Geometry check sheet. Reference: the model listing, model coordinates, mm. A direction names the side the tool comes from. Round coordinates to 2 decimals unless told otherwise and drop trailing zeros. Loops run counter-clockwise (first coordinate to the right, second up) from the corner with the lowest first, then second, coordinate; pieces in that order, holes last. Notation, with made-up numbers: M 78,35.5 L 132,35.5 A17 cw 132,66.5 Z; hole C 82.25,17.5 d1. An arc over 180 degrees is marked long. Use one line per item in the form item = value. Start each with the question number.
1. Material ranges on line 1 (Z direction, x = 10.75, y = -33); line 2 (X direction, y = 35.5, z = 5.75); line 3 (Z direction, x = -11.9, y = 31.75), recorded low to high.
2. Go/stop test with flat-tipped pins: pin 1 (1.5 mm diameter, centred on x = -6, y = -5.5, fed in from -Z); pin 2 (4 mm diameter, centred on y = 24, z = 4.5, fed in from +X). Record where each tip stops, or that it passes through.
3. Cross-section at D-D (z = -9.5). Record the boundary of the cut face in (x, y), then the cut area to 3 significant figures.
4. Cross-section at C-C (y = -19.5). Record the boundary of the cut face in (x, z) (1 decimal).
5. Cross-section at A-A (y = 31.75). Record the boundary of the cut face in (x, z) (1 decimal), then the cut area to 3 significant figures.
6. Draft check along Y on faces 3 (the flat face through (-12, 38.1, 4)), 4 (the cylindrical face through (-2.65, 1.43, 10.5)), 5 (the flat face through (-12, 1, -13.288)). Enter one of: pulls with the +Y half, pulls with the -Y half, needs draft (parallel to the pull), parting line crosses it, or undercut.
7. Cross-section at B-B (z = -4.25). Record the boundary of the cut face in (x, y), then the cut area to 3 significant figures.
8. Set-up check for faces 1 (the cylindrical face through (2.58, 28.65, 10.5)), 2 (the flat face through (-5, -1, 8.937)): record each of +Z, -Z, +X, -X, +Y, -Y from which the full face is reachable in a straight line by a thin tool's end or side.
```python
from build123d import *

# Parameters (mm, degrees)
SKETCH1_W                                 = 76.2
SKETCH1_H                                 = 25.4
BOSS_EXTRUDE1_DEPTH                       = 25.4
SKETCH2_W                                 = 22.225
SKETCH2_H                                 = 22.225
CUT_EXTRUDE1_DEPTH                        = 77.2
FILLET1_R                                 = 1.5875
F_1_4_0_25_DIAMETER_HOLE4_D               = 6.35
F_1_4_0_25_DIAMETER_HOLE4_DEPTH           = 3.175
F_1_4_0_25_DIAMETER_HOLE4_ON_FACE_2_D     = 6.35
F_1_4_0_25_DIAMETER_HOLE4_ON_FACE_2_DEPTH = 3.175
F_3_8_0_375_DIAMETER_HOLE1_D              = 9.525
F_3_8_0_375_DIAMETER_HOLE1_ON_FACE_2_D    = 9.525


with BuildPart() as part:
    # Sketch1 → Boss-Extrude1 (new body)
    with BuildSketch(Plane(origin=(-13.984269616, 0, 0), x_dir=(0, -1, 0), z_dir=(-1, 0, 0))):
        with Locations((0, -0.588041782)):
            Rectangle(SKETCH1_W, SKETCH1_H)
    extrude(amount=-BOSS_EXTRUDE1_DEPTH)

    # Sketch2 → Cut-Extrude1 (cut, through all)
    with BuildSketch(Plane.XZ.offset(38.1)):
        with Locations((0.303230384, -2.175541782)):
            Rectangle(SKETCH2_W, SKETCH2_H)
    extrude(amount=-CUT_EXTRUDE1_DEPTH, mode=Mode.SUBTRACT)

    # Fillet1
    fillet1_edges = [part.edges().sort_by_distance(p)[0] for p in [
        (-13.984269616, 0, 12.111958218),
    ]]
    fillet(fillet1_edges, radius=FILLET1_R)

    # 1/4 (0.25) Diameter Hole4
    with Locations(Plane(origin=(1.890730384, 31.75, 12.111958218), x_dir=(1, 0, 0), z_dir=(0, 0, 1))):
        with Locations((0, 0), (0, -63.5)):
            Hole(F_1_4_0_25_DIAMETER_HOLE4_D / 2, depth=F_1_4_0_25_DIAMETER_HOLE4_DEPTH)

    # 1/4 (0.25) Diameter Hole4 on face 2
    with Locations(Plane(origin=(-13.984269616, 31.75, -3.763041782), x_dir=(0, 0, -1), z_dir=(-1, 0, 0))):
        with Locations((0, 0), (0, 63.5)):
            Hole(F_1_4_0_25_DIAMETER_HOLE4_ON_FACE_2_D / 2, depth=F_1_4_0_25_DIAMETER_HOLE4_ON_FACE_2_DEPTH)

    # 3/8 (0.375) Diameter Hole1 (through all)
    with Locations(Plane(origin=(-13.984269616, 0, -3.763041782), x_dir=(0, 0, -1), z_dir=(-1, 0, 0))):
        with Locations((0, 0)):
            Hole(F_3_8_0_375_DIAMETER_HOLE1_D / 2)

    # 3/8 (0.375) Diameter Hole1 on face 2 (through all)
    with Locations(Plane(origin=(1.890730384, 0, 12.111958218), x_dir=(1, 0, 0), z_dir=(0, 0, 1))):
        with Locations((0, 0)):
            Hole(F_3_8_0_375_DIAMETER_HOLE1_ON_FACE_2_D / 2)


solid = part.part
```
Reported:
q1.line_1 = 8.94 to 12.11
q1.line_2 = -13.98 to -10.81
q1.line_3 = -13.29 to -6.94, -0.59 to 12.11
q2.pin_1 = 8.94
q2.pin_2 = -10.81
q3.outline = M -13.98,-38.1 L -10.81,-38.1 L -10.81,38.1 L -13.98,38.1 Z
q3.area = 242 mm²
q4.outline = M -14,-13.3 L -10.8,-13.3 L -10.8,8.9 L 11.4,8.9 L 11.4,12.1 L -12.4,12.1 A1.6 ccw -14,10.5 Z
q5.outline = M -14,-13.3 L -10.8,-13.3 L -10.8,-6.9 L -14,-6.9 Z; M -14,-0.6 L -10.8,-0.6 L -10.8,8.9 L -1.3,8.9 L -1.3,12.1 L -12.4,12.1 A1.6 ccw -14,10.5 Z; M 5.1,8.9 L 11.4,8.9 L 11.4,12.1 L 5.1,12.1 Z
q5.area = 110 mm²
q6.face_3 = pulls with the +Y half
q6.face_4 = undercut
q6.face_5 = needs draft
q7.outline = M -13.98,-38.1 L -10.81,-38.1 L -10.81,-34.89 L -13.98,-34.89 Z; M -13.98,-28.61 L -10.81,-28.61 L -10.81,-4.74 L -13.98,-4.74 Z; M -13.98,4.74 L -10.81,4.74 L -10.81,28.61 L -13.98,28.61 Z; M -13.98,34.89 L -10.81,34.89 L -10.81,38.1 L -13.98,38.1 Z
q7.area = 172 mm²
q8.face_1 = +Z, -Z
q8.face_2 = -Z, +X, +Y, -Y
